Input: part model. Units: mm. Frame: model coordinates. A direction names the side the tool comes from. Give positions to 0.01 mm unless a question says otherwise; leave off trailing zeros. Loops run counter-clockwise (first coordinate to the right, second up) from the corner with the lowest first, then second, coordinate; pieces in that order, holes last. Notation, with made-up numbers: (12, 68.25) - (41, 68.25) arc R12 cw to (41, 91.25) - close; hole circle Ø10 at (-10, -23). An arc over 180 degrees is marked (long way). One line per item, written item: value.
from build123d import *

# Parameters (mm, degrees)
F0_R     = 22.5
F1_DEPTH = 10
F2_R     = 11
F3_DEPTH = 11
F5_D     = 8.2
F7_D     = 5.3
F8_R     = 2.25
F9_DEPTH = 50


with BuildPart() as f1:
    # F0 (on Top) → F1 (new body)
    with BuildSketch(Plane.XY):
        Circle(F0_R)
    extrude(amount=F1_DEPTH)

    # F2 (on face) → F3 (join)
    with BuildSketch(Plane.XY.offset(10)):
        Circle(F2_R)
    extrude(amount=F3_DEPTH)

    # F5 (through all)
    with Locations(Plane.XY.offset(21)):
        with Locations((0, 0)):
            Hole(F5_D / 2)

    # F7 (through all)
    with Locations(Plane.XY.offset(10)):
        with Locations((0, 17), (14.722432, 8.5), (14.722432, -8.5), (0, -17), (-14.722432, -8.5), (-14.722432, 8.5)):
            Hole(F7_D / 2)

    # F8 (on Right) → F9 (cut, symmetric)
    with BuildSketch(Plane.YZ):
        with Locations((0, 17)):
            Circle(F8_R)
    extrude(amount=F9_DEPTH, both=True, mode=Mode.SUBTRACT)


solid = f1.part
Item 1: Section B-B, the plane y = -8.5. Output: boundary loops of the cut face in (x, z).
Verdict:
outline: (-20.83, 0) - (-17.37, 0) - (-17.37, 10) - (-20.83, 10) - close; (-12.07, 0) - (12.07, 0) - (12.07, 10) - (6.98, 10) - (6.98, 21) - (-6.98, 21) - (-6.98, 10) - (-12.07, 10) - close; (17.37, 0) - (20.83, 0) - (20.83, 10) - (17.37, 10) - close
Item 2: Material intervals for L1, parallel to Y at x = 14, z = 7.5; L2, parallel to X at y = 10, z = 2; L3, parallel to Y at x = 13, z = 9.5, sorted ascending.
Verdict:
L1: y = -17.61 to -11.05, -5.95 to 5.95, 11.05 to 17.61
L2: x = -20.16 to -16.91, -12.54 to 12.54, 16.91 to 20.16
L3: y = -18.36 to -10.51, -6.49 to 6.49, 10.51 to 18.36
Item 3: Section A-A, the plane x = 0. Output: boundary loops of the cut face in (y, z), and give its area (3 significant figures).
Verdict:
outline: (-22.5, 0) - (-19.65, 0) - (-19.65, 10) - (-22.5, 10) - close; (-14.35, 0) - (-4.1, 0) - (-4.1, 21) - (-11, 21) - (-11, 10) - (-14.35, 10) - close; (4.1, 0) - (14.35, 0) - (14.35, 10) - (11, 10) - (11, 21) - (4.1, 21) - close; (19.65, 0) - (22.5, 0) - (22.5, 10) - (19.65, 10) - close
area: 414 mm^2
Item 4: Pin query (flat end, axial travel): P1, Ø8.5, axis at x = 14.72, y = -8.5, coming from the +Z side; P2, Ø1.5, axis at y = 10, z = 7.5, coming from the +X side; P3, Ø1.5, axis at y = -14, z = 6, coming from the +X side. Return the tip coordinate at first contact, or that it passes through.
Verdict:
P1: stops at z = 10
P2: stops at x = 20.51
P3: stops at x = 18.18
Item 5: Section D-D, the plane x = 16. Output: boundary loops of the cut face in (y, z).
Verdict:
outline: (-15.82, 0) - (-10.82, 0) - (-10.82, 10) - (-15.82, 10) - close; (-6.18, 0) - (6.18, 0) - (6.18, 10) - (-6.18, 10) - close; (10.82, 0) - (15.82, 0) - (15.82, 10) - (10.82, 10) - close
Item 6: Section C-C, the plane z = 3. Output: boundary loops of the cut face in (x, y).
Verdict:
outline: circle Ø45 at (0, 0); hole circle Ø5.3 at (-14.72, -8.5); hole circle Ø5.3 at (-14.72, 8.5); hole circle Ø8.2 at (0, 0); hole circle Ø5.3 at (0, -17); hole circle Ø5.3 at (0, 17); hole circle Ø5.3 at (14.72, -8.5); hole circle Ø5.3 at (14.72, 8.5)
Item 7: Draft query along Y for faces 3 (the face through (5, 0, 0)), 4 (the face through (10.382, -19.961, 4.93)), 5 (the face through (-1.425, 19.234, 4.93)). Return one class per face: pulls with the +Y half, pulls with the -Y half, needs draft (parallel to the pull), parting line crosses it, or undercut.
Verdict:
face 3: needs draft
face 4: parting line crosses it
face 5: undercut
Item 8: Access query for faces 1 (the face through (0.57, -19.59, 4.93)), 2 (the face through (10.161, -4.213, 15.423)). Directions: +Z, -Z, +X, -X, +Y, -Y. A direction counts if a zero-diameter tool reaches every point of the face in a straight line with its end or side. Return the directions, or none.
Verdict:
face 1: +Z, -Z
face 2: +Z
